```python
from build123d import *

# Parameters (mm, degrees)
SKETCH1_R           = 5.000000033
SKETCH1_R_2         = 3
BOSS_EXTRUDE1_DEPTH = 3
BOSS_EXTRUDE2_DEPTH = 2


with BuildPart() as part:
    # Sketch1 → Boss-Extrude1 (new body)
    with BuildSketch(Plane(origin=(0, 0, 0), x_dir=(1, 0, 0), z_dir=(0, 1, 0))):
        Circle(SKETCH1_R)
        Circle(SKETCH1_R_2, mode=Mode.SUBTRACT)
    extrude(amount=BOSS_EXTRUDE1_DEPTH)

    # Sketch2 → Boss-Extrude2 (add)
    with BuildSketch(Plane(origin=(0, 3, 0), x_dir=(1, 0, 0), z_dir=(0, 1, 0))):
        with BuildLine():
            Line((4.416654416, 2.343750007), (1.104163597, 8.585937596))
            ThreePointArc((1.104163597, 8.585937596), (0, 9.250000098), (-1.104163597, 8.585937596))
            Line((-1.104163597, 8.585937596), (-4.416654416, 2.343750007))
            ThreePointArc((-4.416654416, 2.343750007), (0, -5.000000033), (4.416654416, 2.343750007))
        make_face()
    extrude(amount=BOSS_EXTRUDE2_DEPTH)


solid = part.part
```
Could you check a few things on this model? Use its own coordinates, in mm. A direction names the side the tool comes from. Give positions to 0.01 mm unless a question says otherwise; leave off trailing zeros. Write each loop counter-clockwise with the first axis right and the second up, starting at its lowest first coordinate (ties: lowest second). Pieces come first, ordered by that corner, then holes. Notation, with made-up numbers: (70.5, -9.75) - (128.5, -9.75) arc R25 cw to (128.5, 22.25) - close; hole circle Ø2 at (-26.5, 32). An arc over 180 degrees is marked (long way). One line per item, written item: value. Start each with the question number.
Item 1: Imagine slicing it at D-D, the plane y = 4. List the corners of the cut face in (x, z) for me, and give its area (3 significant figures).
Item 2: Imagine slicing it at C-C, the plane z = 0. List the corners of the cut face in (x, y) for me, and give its area (3 significant figures).
Item 3: Imagine slicing it at B-B, the plane y = 1.95. List the corners of the cut face in (x, z) for me, and give its area (3 significant figures).
Item 4: Which directions (+Z, -Z, +X, -X, +Y, -Y) give clear straight access to the entire face, cutting with the end or side of a thin tool? Please do faces 4 (the face through (0, 3, 0)), 5 (the face through (0.02, 3.99, -9.25)).
Item 5: If we mould it in two halves opening along Z, with no side actions, what happens to faces 1 (the face through (-0.1, 0, 3.3)), 2 (the face through (-2.737, 3.986, -5.509)), 3 (the face through (-3, 1, 0))? For each: +Z half, -Z half, draft (parallel to the pull), parting line (faces both ways), or undercut.
Item 6: Please list where these lines run through material, in increasing order: line 1 (X direction, y = 1.2, z = 0); line 2 (Y direction, x = 0.5, z = 0.25). Write a range as from..to.
Item 7: Imagine slicing it at A-A, the plane x = 0. List the corners of the cut face in (y, z) for me.
Item 8: I'm going to push flat-ended pins straight in: pin 1 (1 mm diameter, centred on x = 1, y = 3, fed in from +Z); pin 2 (1.8 mm diameter, centred on x = 0.5, z = -0.5, fed in from -Y). Where does each tip first touch, or does it pass through?
Geometry says:
1. outline: (-4.42, -2.34) - (-1.1, -8.59) arc R1.25 ccw to (1.1, -8.59) - (4.42, -2.34) arc R5 ccw (long way) to start
1. area: 97.3 mm^2
2. outline: (-5, 0) - (-3, 0) - (-3, 3) - (3, 3) - (3, 0) - (5, 0) - (5, 5) - (-5, 5) - close
2. area: 32.0 mm^2
3. outline: circle Ø10 at (0, 0); hole circle Ø6 at (0, 0)
3. area: 50.3 mm^2
4. face 4: -Y
4. face 5: -Z, +Y, -Y
5. face 1: draft
5. face 2: -Z half
5. face 3: undercut
6. line 1: -5..-3, 3..5
6. line 2: 3..5
7. outline: (0, -5) - (3, -5) - (3, -9.25) - (5, -9.25) - (5, 5) - (0, 5) - (0, 3) - (3, 3) - (3, -3) - (0, -3) - close
8. pin 1: z = 4.97
8. pin 2: y = 3
